from build123d import *

# Parameters (mm, degrees)
CHAMFER1_SIZE   = 0.75
CHAMFER1_SIZE_2 = 0.597274803


with BuildPart() as part:
    # Sketch1 → Revolve1 (revolve)
    with BuildSketch(Plane.XY):
        Polygon((-4.2, -12.5), (-4.25, -12.5), (-4.25, -20), (-20, -25), (0, -25), (0, 25), (-4, 25), (-4, 17.5), (-4.05, 17.5), (-4.05, 10), (-4.1, 10), (-4.1, 2.5), (-4.15, 2.5), (-4.15, -5), (-4.2, -5), align=None)
    revolve(axis=Axis((0, 37.271191626, 0), (0, -1, 0)))

    # Chamfer1
    # the kernel refuses this chamfer: 0.75, 0.597274803 mm, written as the material it adds along each edge
    with BuildSketch(Plane(origin=(0, 10, 0), x_dir=(-1, 0, 0), z_dir=(0, 0, 1))) as chamfer1_piece_1_section:
        Polygon((4.05, -CHAMFER1_SIZE), (4.05 + CHAMFER1_SIZE, 0), (4.05, 0), align=None)
    chamfer1_piece_1 = revolve(axis=Axis((0, 10, 0), (0, -1, 0)), mode=Mode.PRIVATE)
    chamfer1_piece_1 = chamfer1_piece_1 & Plane(origin=(0, 10.727876621, 0), x_dir=(-1, 0, 0), z_dir=(0, -1, 0)) * Cylinder(4.1, 20, mode=Mode.PRIVATE)
    add(chamfer1_piece_1)
    # the kernel refuses this chamfer: 0.75, 0.597274803 mm, written as the material it takes off along each edge
    with BuildSketch(Plane(origin=(0, 25, 0), x_dir=(-1, 0, 0), z_dir=(0, 0, 1))) as chamfer1_2_piece_1:
        Polygon((4, CHAMFER1_SIZE), (4 - CHAMFER1_SIZE, 0), (4, 0), align=None)
    revolve(axis=Axis((0, 25, 0), (0, -1, 0)), mode=Mode.SUBTRACT)
    with BuildSketch(Plane(origin=(0, 17.5, 0), x_dir=(-1, 0, 0), z_dir=(0, 0, 1))) as chamfer1_2_piece_2_section:
        Polygon((4.05, CHAMFER1_SIZE), (4.05 - CHAMFER1_SIZE, 0), (4.05, 0), align=None)
    chamfer1_2_piece_2 = revolve(axis=Axis((0, 17.5, 0), (0, -1, 0)), mode=Mode.PRIVATE)
    chamfer1_2_piece_2 = chamfer1_2_piece_2 - Plane(origin=(0, 16.772104401, 0), x_dir=(-1, 0, 0), z_dir=(0, -1, 0)) * Cylinder(4, 17, mode=Mode.PRIVATE)
    add(chamfer1_2_piece_2, mode=Mode.SUBTRACT)
    with BuildSketch(Plane(origin=(0, -25, 0), x_dir=(-1, 0, 0), z_dir=(0, 0, 1))) as chamfer1_2_piece_3:
        Polygon((20 - CHAMFER1_SIZE_2 * 0.953124266375, -CHAMFER1_SIZE_2 * 0.302579132183), (20 - CHAMFER1_SIZE, 0), (20, 0), align=None)
    revolve(axis=Axis((0, -25, 0), (0, -1, 0)), mode=Mode.SUBTRACT)


solid = part.part
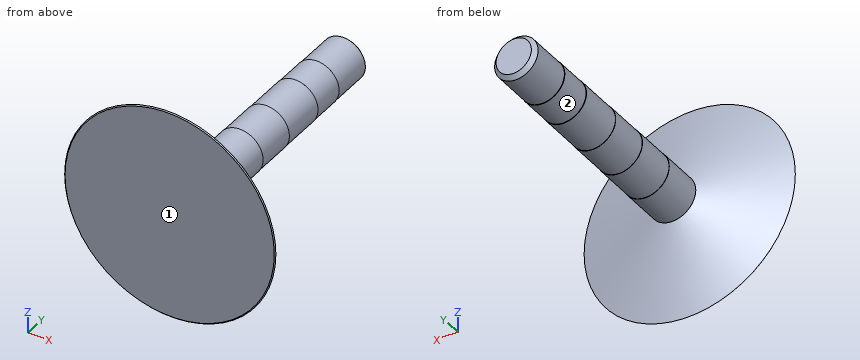
Could you check a few things on this model? Use its own coordinates, in mm. Face numbers are marked on the shaded views. A direction names the side the tool comes from. Coordinates: 2 decimals unless noted, no trailing zeros. Write each loop counter-clockwise with the first axis right and the second up, starting at its lowest first coordinate (ties: lowest second). Pieces come first, ordered by that corner, then holes. Notation, with made-up numbers: (15.25, -24) - (26.25, -24) arc R23 ccw to (26.25, 12) - close; hole circle Ø6 at (33.25, 19.5). An arc over 180 degrees is marked (long way). Put each result on its own line as item: value. Start each with the question number.
Q1. I want a section at C-C on y = 16. Write out the boundary of the cut face in (x, z), plus the area to 3 significant figures.
Q2. I want a section at D-D on y = -13.5. Write out the boundary of the cut face in (x, z).
Q3. Please list where these lines run through material, in increasing order: L1, parallel to X at y = 19.5, z = 1.5; L2, parallel to Y at x = -6, z = -5; L3, parallel to Y at x = 0.5, z = -14.5.
Q4. I'm going to push flat-ended pins straight in: P1, Ø1.5, axis at x = 3.5, z = 2, coming from the +Y side; P2, Ø5, axis at y = 2, z = 6, coming from the +X side; P3, Ø3, axis at x = 14, z = -2.5, coming from the +Y side. Where does each tip first touch, or does it pass through?
Q5. Which directions (+Z, -Z, +X, -X, +Y, -Y) give clear straight access to the entire face, cutting with the end or side of a thin tool? Please do the marked faces 1 and 2.
Checks:
1. outline: circle Ø8.1 at (0, 0)
1. area: 51.5 mm²
2. outline: circle Ø8.5 at (0, 0)
3. L1: -3.71 to 3.71
3. L2: -25 to -21.13
3. L3: -25 to -23.26
4. P1: y = 24.97
4. P2: x = 2.23
4. P3: y = -22.69
5. face 1: +Z, -Z, +X, -X, -Y
5. face 2: +Y
